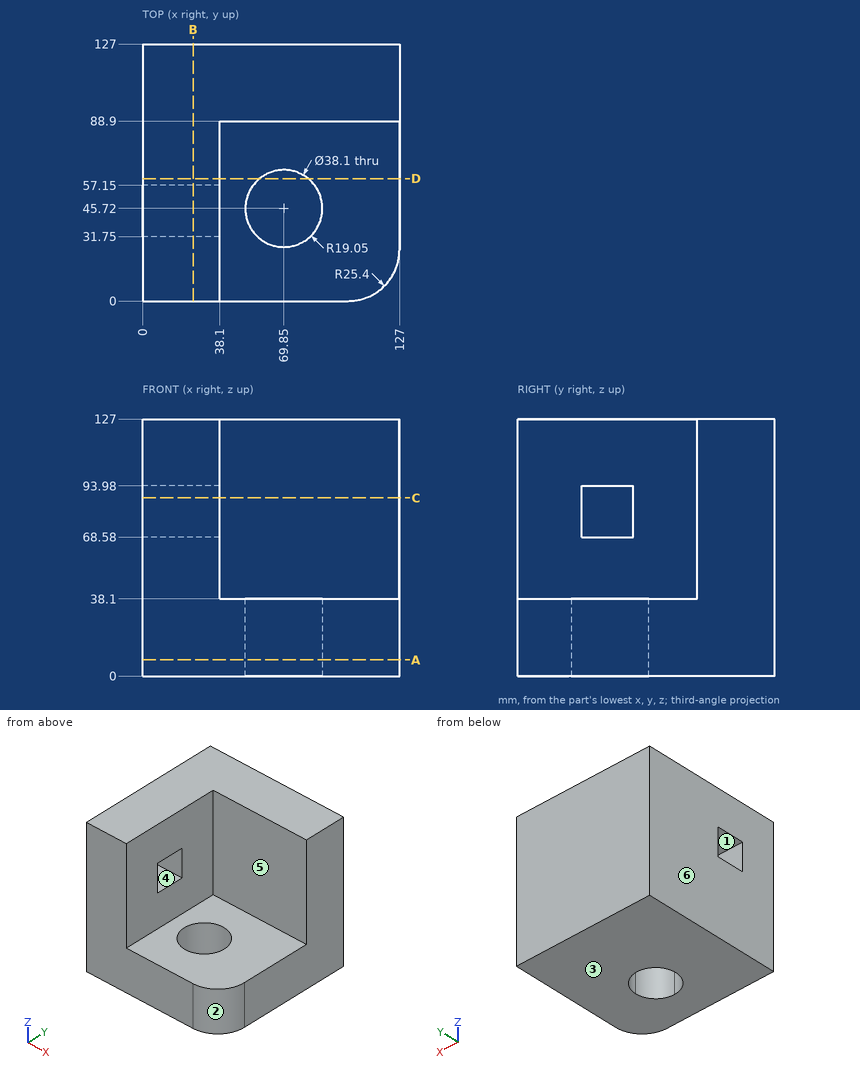
Input: dimensioned drawing with shaded views. Units: mm. Origin: part minimum x, y, z. A direction names the side the tool comes from. Coordinates: 2 decimals unless noted, no trailing zeros. Write each loop counter-clockwise with the first axis right and the second up, starting at its lowest first coordinate (ties: lowest second). Pieces come first, ordered by that corner, then holes. Notation, with made-up numbers: M 15,41.5 L 56,41.5 A29 ccw 56,79.5 Z; hole C 31.25,53 d4. An arc over 180 degrees is marked long. Answer as a JSON object with one key per item and string values. Group by question number.
(1) Ray query, line 1 along X through (y, z) = (45.72, 13.5); line 2 along Y through (x, z) = (69, 27); line 3 along Z through (x, y) = (24.5, 48). Return the intervals inside material, ascending. Write a range as [from, to].
(2) Section D-D on y = 60.5. Output: boundary loops of the cut face in (x, z).
(3) Section A-A on z = 8. Output: boundary loops of the cut face in (x, y).
(4) Section C-C on z = 88. Output: boundary loops of the cut face in (x, y).
(5) Section B-B on x = 25. Output: boundary loops of the cut face in (y, z).
(6) Mould query, pull axis Y, two halves, no side actions, for the marked faces 1, 2 and 3. Classes: pulls with the +Y half, pulls with the -Y half, needs draft (parallel to the pull), parting line crosses it, or undercut.
(7) Set-up query: the marked faces 4, 5 and 6. Return all of +Z, -Z, +X, -X, +Y, -Y with unobstructed straight access to the full face (end or side cutting, diameter ignored); none if empty.
(8) Contact query for a flat-ended pin moving along its axis: P1, Ø3, axis at x = 92.5, z = 59, coming from the -Y side. Output: stop coordinate, or through.
Result set:
{
 "1": {"line 1": "x = [0, 50.8], [88.9, 127]", "line 2": "y = [0, 26.69], [64.75, 127]", "line 3": "z = [0, 68.58], [93.98, 127]"},
 "2": {"outline": "M 0,0 L 57.83,0 L 57.83,38.1 L 38.1,38.1 L 38.1,127 L 0,127 Z; M 81.87,0 L 127,0 L 127,38.1 L 81.87,38.1 Z"},
 "3": {"outline": "M 0,0 L 101.6,0 A25.4 ccw 127,25.4 L 127,127 L 0,127 Z; hole C 69.85,45.72 d38.1"},
 "4": {"outline": "M 0,0 L 38.1,0 L 38.1,31.75 L 0,31.75 Z; M 0,57.15 L 38.1,57.15 L 38.1,88.9 L 127,88.9 L 127,127 L 0,127 Z"},
 "5": {"outline": "M 0,0 L 127,0 L 127,127 L 0,127 Z; hole M 31.75,68.58 L 57.15,68.58 L 57.15,93.98 L 31.75,93.98 Z"},
 "6": {"face 1": "undercut", "face 2": "pulls with the -Y half", "face 3": "needs draft"},
 "7": {"face 4": "+X, -X", "face 5": "+Z, +X, -Y", "face 6": "+Z, -Z, -X, +Y, -Y"},
 "8": {"P1": "stops at y = 88.9"}
}
